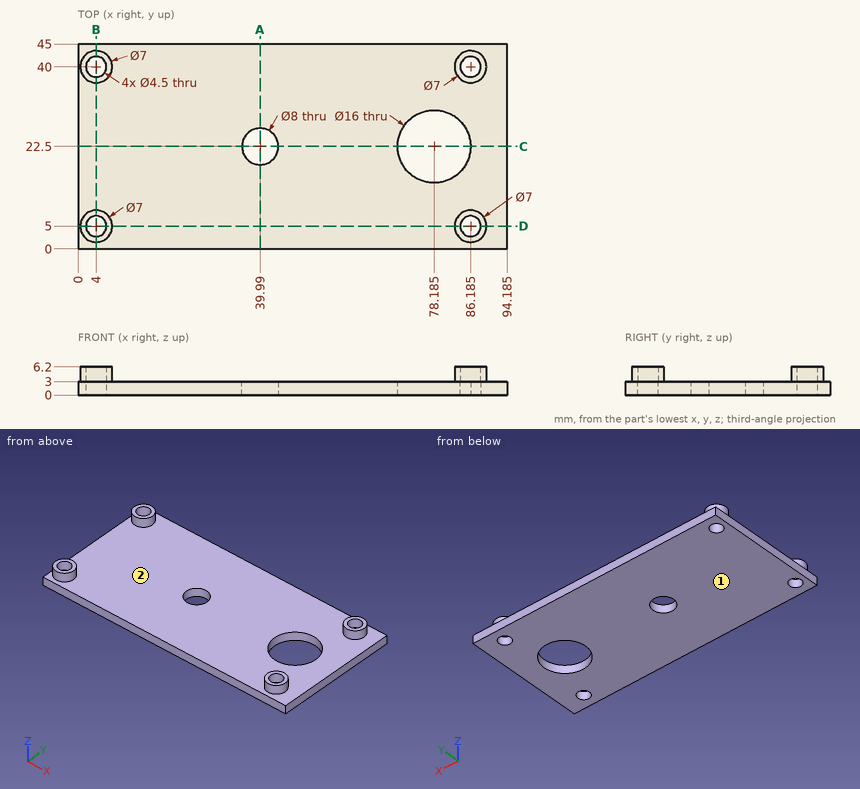
Drawing for the job (mm, zero at the part's lowest x, y, z). A direction names the side the tool comes from. Coordinates: 2 decimals unless noted, no trailing zeros. Loops run counter-clockwise (first coordinate to the right, second up) from the corner with the lowest first, then second, coordinate; pieces in that order, holes last. Notation, with made-up numbers: (-1.5, 49.25) - (15.5, 49.25) arc R19 cw to (15.5, 56.25) - close; hole circle Ø10 at (52.25, 50.25). An arc over 180 degrees is marked (long way). Use CSV: the item, a comma, the result in double quotes. Start each with the question number.
Q1. 3-axis set-ups, long thin cutter, end or side, ignore diameter. For the marked faces 1 and 2: which of +Z, -Z, +X, -X, +Y, -Y reach the whole face in a straight line?
Q2. Probe probe 1 along Y at (x, z) = (4, 5.35); probe 2 along Y at (x, z) = (4, 1.75); probe 3 along X at (y, z) = (22, 2.75) (3 decimals). List the from-to ranges inside material, lowest first. Write a range as from..to.
Q3. Cut at D-D, the plane y = 5. List the corners of the cut face in (x, z) (3 decimals).
Q4. Drop a flat-ended pin along its axis: P1, Ø4, axis at x = 86.185, y = 5, coming from the -Z side. Give the stop position or say it passes through.
Q5. Cut at A-A, the plane x = 39.99. List the corners of the cut face in (y, z), then the cut area to 3 significant figures.
Q6. Cut at C-C, the plane y = 22.5. List the corners of the cut face in (x, z) (3 decimals), then the cut area to 3 significant figures.
Q7. Cut at B-B, the plane x = 4. List the corners of the cut face in (y, z), then the cut area to 3 significant figures.
Here are the results:
1,face 1,"-Z, +X, -X, +Y, -Y"
1,face 2,"+Z"
2,probe 1,"1.5..2.75, 7.25..8.5, 36.5..37.75, 42.25..43.5"
2,probe 2,"0..2.75, 7.25..37.75, 42.25..45"
2,probe 3,"0..36.021, 43.959..70.201, 86.169..94.185"
3,outline,"(0, 0) - (1.75, 0) - (1.75, 6.2) - (0.5, 6.2) - (0.5, 3) - (0, 3) - close; (6.25, 0) - (83.935, 0) - (83.935, 6.2) - (82.685, 6.2) - (82.685, 3) - (7.5, 3) - (7.5, 6.2) - (6.25, 6.2) - close; (88.435, 0) - (94.185, 0) - (94.185, 3) - (89.685, 3) - (89.685, 6.2) - (88.435, 6.2) - close"
4,P1,"through"
5,outline,"(0, 0) - (18.5, 0) - (18.5, 3) - (0, 3) - close; (26.5, 0) - (45, 0) - (45, 3) - (26.5, 3) - close"
5,area,"111 mm2"
6,outline,"(0, 0) - (35.99, 0) - (35.99, 3) - (0, 3) - close; (43.99, 0) - (70.185, 0) - (70.185, 3) - (43.99, 3) - close; (86.185, 0) - (94.185, 0) - (94.185, 3) - (86.185, 3) - close"
6,area,"211 mm2"
7,outline,"(0, 0) - (2.75, 0) - (2.75, 6.2) - (1.5, 6.2) - (1.5, 3) - (0, 3) - close; (7.25, 0) - (37.75, 0) - (37.75, 6.2) - (36.5, 6.2) - (36.5, 3) - (8.5, 3) - (8.5, 6.2) - (7.25, 6.2) - close; (42.25, 0) - (45, 0) - (45, 3) - (43.5, 3) - (43.5, 6.2) - (42.25, 6.2) - close"
7,area,"124 mm2"
